```python
from build123d import *


with BuildPart() as part:
    # Sketch1 → Revolve1 (revolve)
    with BuildSketch(Plane.XY):
        with BuildLine():
            Line((0, 0), (0, 4.8006))
            Line((0, 4.8006), (0.75565, 5.55625))
            Line((0.75565, 5.55625), (4.660293864, 5.55625))
            Line((4.660293864, 5.55625), (5.418103291, 4.804192648))
            ThreePointArc((5.418103291, 4.804192648), (5.676923575, 4.6323221), (5.9817, 4.572))
            Line((5.9817, 4.572), (7.1501, 4.572))
            ThreePointArc((7.1501, 4.572), (7.715856136, 4.806343864), (7.9502, 5.3721))
            Line((7.9502, 5.3721), (7.9502, 5.53085))
            Line((7.9502, 5.53085), (9.525, 5.53085))
            Line((9.525, 5.53085), (9.525, 0))
            Line((9.525, 0), (0, 0))
        make_face()
    revolve(axis=Axis((9.525, 0, 0), (-1, 0, 0)))

    # Sketch2 → Revolve2 (revolve)
    with BuildSketch(Plane.XY):
        Polygon((9.525, 0), (9.525, 7.0485), (10.287, 7.8105), (25.1206, 7.8105), (25.3746, 7.5565), (25.3746, 6.63575), (26.0096, 6.63575), (26.6446, 7.27075), (28.8544, 7.27075), (29.3624, 6.76275), (29.3624, 0), align=None)
    revolve(axis=Axis((29.3624, 0, 0), (-1, 0, 0)))

    # Sketch3 → Cut-Revolve1 (revolve, cut)
    with BuildSketch(Plane.XY):
        Polygon((0, 0), (0, 2.921), (0.508, 2.413), (29.3624, 2.413), (29.3624, 0), align=None)
    revolve(axis=Axis((29.3624, 0, 0), (-1, 0, 0)), mode=Mode.SUBTRACT)

    # Sketch4 → Cut-Revolve2 (revolve, cut)
    with BuildSketch(Plane(origin=(0, 0, 0), x_dir=(1, 0, 0), z_dir=(0, 1, 0))):
        Polygon((19.05, 1.016), (21.03374, 1.016), (21.03374, -6.36524), (21.463, -6.7945), (23.0124, -6.7945), (23.0124, -7.8105), (19.05, -7.8105), align=None)
    revolve(axis=Axis((19.05, 0, 7.8105), (0, 0, -1)), mode=Mode.SUBTRACT)

    # Sketch5 → Revolve3 (revolve)
    with BuildSketch(Plane.XY):
        with BuildLine():
            Line((25.3746, 7.186143808), (25.3746, 6.38175))
            Line((25.3746, 6.38175), (26.0096, 6.38175))
            Line((26.0096, 6.38175), (26.0096, 6.63575))
            Line((26.0096, 6.63575), (25.6921, 6.63575))
            Line((25.6921, 6.63575), (25.491639755, 6.836210245))
            ThreePointArc((25.491639755, 6.836210245), (25.454442316, 6.926012806), (25.491639755, 7.015815367))
            Line((25.491639755, 7.015815367), (26.202156192, 7.726331804))
            Line((26.202156192, 7.726331804), (26.202156192, 7.8105))
            Line((26.202156192, 7.8105), (25.998956192, 7.8105))
            Line((25.998956192, 7.8105), (25.3746, 7.186143808))
        make_face()
    revolve(axis=Axis((26.0096, 0, 0), (-1, 0, 0)))


solid = part.part
```
Could you check a few things on this model? Use its own coordinates, in mm. A direction names the side the tool comes from. Round coordinates to 2 decimals unless told otherwise and drop trailing zeros. Loops run counter-clockwise (first coordinate to the right, second up) from the corner with the lowest first, then second, coordinate; pieces in that order, holes last.
Q1. I want a section at D-D (x = 22.5). Write out the boundary of the cut face in (y, z), and give its area (3 significant figures).
Q2. For P1, Ø4, axis at x = 17, z = 4.5, coming from the -Y side; P2, Ø4, axis at x = 21, y = 1, coming from the +Z side; P3, Ø5, axis at y = 5.5, z = 5, coming from the -X side, each with a flat end and sliding along its axis, tell me the tip position at first contact or that it passes through.
Q3. I want a section at C-C (y = 0). Give the number of separate pieces and of enclosed holes in the cut face, and give its area (3 significant figures).
Q4. Please list where these lines run through material, in increasing order: L1, parallel to Y at x = 11, z = 0; L2, parallel to Y at x = 19.05, z = 2.85; L3, parallel to X at y = 0, z = 3.95.
Q5. Thinking about a two-plate mould opening in Y: for faces 3 (the cylindrical face through (17.48, 1.21, 3.9)), 4 (the flat face through (9.525, -3, 5)), 5 (the cylindrical face through (2.74, 5.3, -1.67)), 6 (the cylindrical face through (15.137, -0.314, -2.392)), which applies, pulls with the +Y half, pulls with the -Y half, needs draft (parallel to the pull), parting line crosses it, or undercut?
Q6. On a 3-axis mill with a long thin cutter (end or side, diameter ignored), from which of +Z, -Z, +X, -X, +Y, -Y can I reach the whole of each face in a straight line? I mean faces 1 (the flat face through (0, 0.1, 3.1)), 2 (the cylindrical face through (6.574, -0.991, 4.463)). Say none if no direction works.
Q7. I want a section at B-B (x = 19.05). Write out the boundary of the cut face in (y, z), and give its area (3 significant figures).
Q8. I want a section at A-A (x = 8.25). Write out the boundary of the cut face in (y, z), and give its area (3 significant figures).
Answer below:
1. outline: (-1.95, 6.79) - (-1.95, 7.56) arc R7.81 ccw (long way) to (1.95, 7.56) - (1.95, 6.79) - close; hole circle Ø4.83 at (0, 0)
1. area: 170 mm2
2. P1: stops at y = -7.4
2. P2: stops at z = 7.79
2. P3: stops at x = 0.13
3. separate pieces: 3
3. enclosed holes: 0
3. area: 236 mm2
4. L1: y = -7.81 to -2.41, 2.41 to 7.81
4. L2: y = -7.27 to -1.98, 1.98 to 7.27
4. L3: x = 0 to 17.07, 21.03 to 29.36
5. face 3: undercut
5. face 4: needs draft
5. face 5: parting line crosses it
5. face 6: undercut
6. face 1: +Z, -Z, -X, +Y, -Y
6. face 2: none
7. outline: (-3.85, 6.79) arc R7.81 ccw (long way) to (3.85, 6.79) - (2.41, 6.79) - (1.98, 6.37) - (1.98, 1.37) arc R2.41 cw (long way) to (-1.98, 1.37) - (-1.98, 6.37) - (-2.41, 6.79) - close
7. area: 149 mm2
8. outline: circle Ø11.06 at (0, 0); hole circle Ø4.83 at (0, 0)
8. area: 77.8 mm2
